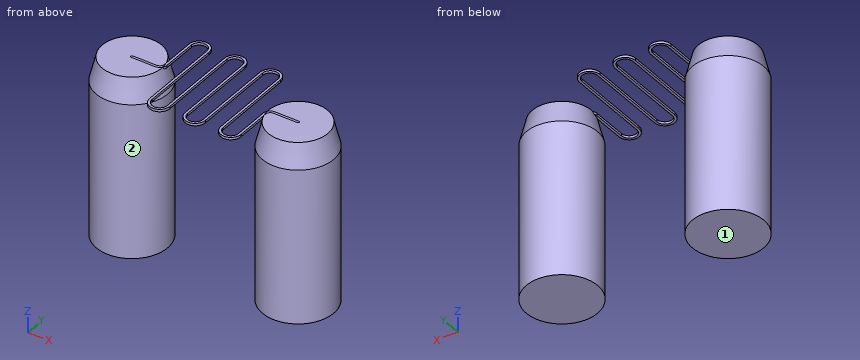
```python
from build123d import *
from build123d.topology import SkipClean

# Parameters (mm, degrees)
BOSS_EXTRUDE1_DEPTH = 0.4


with BuildPart() as part:
    # Sketch2 → Boss-Extrude1 (new body)
    with BuildSketch(Plane.XY):
        with BuildLine():
            Line((-17.5, -0.2), (-13.5, -0.2))
            ThreePointArc((-13.5, -0.2), (-12.651471863, 0.151471863), (-12.3, 1))
            Line((-12.3, 1), (-12.3, 7))
            ThreePointArc((-12.3, 7), (-11, 8.3), (-9.7, 7))
            Line((-9.7, 7), (-9.7, 0))
            Line((-9.7, 0), (-9.7, -7))
            ThreePointArc((-9.7, -7), (-8, -8.7), (-6.3, -7))
            Line((-6.3, -7), (-6.3, 0))
            Line((-6.3, 0), (-6.3, 7))
            ThreePointArc((-6.3, 7), (-5, 8.3), (-3.7, 7))
            Line((-3.7, 7), (-3.7, 0))
            Line((-3.7, 0), (-3.7, -7))
            ThreePointArc((-3.7, -7), (-2, -8.7), (-0.3, -7))
            Line((-0.3, -7), (-0.3, 0))
            Line((-0.3, 0), (-0.3, 7))
            ThreePointArc((-0.3, 7), (1, 8.3), (2.3, 7))
            Line((2.3, 7), (2.3, 0))
            Line((2.3, 0), (2.3, -7))
            ThreePointArc((2.3, -7), (4, -8.7), (5.7, -7))
            Line((5.7, -7), (5.7, -1))
            ThreePointArc((5.7, -1), (5.934314575, -0.434314575), (6.5, -0.2))
            Line((6.5, -0.2), (10.5, -0.2))
            ThreePointArc((10.5, -0.2), (10.7, 0), (10.5, 0.2))
            Line((10.5, 0.2), (6.5, 0.2))
            ThreePointArc((6.5, 0.2), (5.651471863, -0.151471863), (5.3, -1))
            Line((5.3, -1), (5.3, -7))
            ThreePointArc((5.3, -7), (4, -8.3), (2.7, -7))
            Line((2.7, -7), (2.7, 0))
            Line((2.7, 0), (2.7, 7))
            ThreePointArc((2.7, 7), (1, 8.7), (-0.7, 7))
            Line((-0.7, 7), (-0.7, 0))
            Line((-0.7, 0), (-0.7, -7))
            ThreePointArc((-0.7, -7), (-2, -8.3), (-3.3, -7))
            Line((-3.3, -7), (-3.3, 0))
            Line((-3.3, 0), (-3.3, 7))
            ThreePointArc((-3.3, 7), (-5, 8.7), (-6.7, 7))
            Line((-6.7, 7), (-6.7, 0))
            Line((-6.7, 0), (-6.7, -7))
            ThreePointArc((-6.7, -7), (-8, -8.3), (-9.3, -7))
            Line((-9.3, -7), (-9.3, 0))
            Line((-9.3, 0), (-9.3, 7))
            ThreePointArc((-9.3, 7), (-11, 8.7), (-12.7, 7))
            Line((-12.7, 7), (-12.7, 1))
            ThreePointArc((-12.7, 1), (-12.934314575, 0.434314575), (-13.5, 0.2))
            Line((-13.5, 0.2), (-17.5, 0.2))
            ThreePointArc((-17.5, 0.2), (-17.7, 0), (-17.5, -0.2))
        make_face()
    extrude(amount=BOSS_EXTRUDE1_DEPTH)

    # Sketch3 → Revolve1 (revolve)
    with SkipClean():  # the faces are left unmerged after this step: merging them gives an invalid solid
        with BuildSketch(Plane(origin=(0, 0, 0), x_dir=(-1, 0, 0), z_dir=(0, -1, 0)), mode=Mode.PRIVATE) as revolve1_sk:
            Polygon((17.5, -0.4), (22.5, -0.4), (23.5, 3.6), (23.5, 29.6), (17.5, 29.6), align=None)
        revolve(revolve1_sk.sketch.rotate(Axis((-17.5, 0, 0.4), (0, 0, -1)), 160.250078189), axis=Axis((-17.5, 0, 0.4), (0, 0, -1)))

    # Sketch4 → Revolve2 (revolve)
    with SkipClean():  # the faces are left unmerged after this step: merging them gives an invalid solid
        with BuildSketch(Plane(origin=(0, 0, 0), x_dir=(-1, 0, 0), z_dir=(0, -1, 0)), mode=Mode.PRIVATE) as revolve2_sk:
            Polygon((-10.5, -0.4), (-15.5, -0.4), (-16.5, 3.6), (-16.5, 29.6), (-10.5, 29.6), align=None)
        revolve(revolve2_sk.sketch.rotate(Axis((10.5, 0, 0.4), (0, 0, -1)), 176.315074658), axis=Axis((10.5, 0, 0.4), (0, 0, -1)))


solid = part.part
```
Design review of the part built by this model. Coordinates are the model's own, in mm. Face numbers are marked on the shaded views. Give positions to 0.01 mm unless a question says otherwise; leave off trailing zeros. Loops run counter-clockwise (first coordinate to the right, second up) from the corner with the lowest first, then second, coordinate; pieces in that order, holes last. Notation, with made-up numbers: M -34,22.25 L 19,22.25 A29 cw 19,47.25 Z; hole C 59.25,-35 d11. An arc over 180 degrees is marked long. Return JSON: item names as keys, results as strings. Group by question number.
Item 1: We need section A-A (x = 1). Give the boundary of the cut face in (y, z).
Item 2: Insertion check: pin 1 Ø3 at (x, y) = (-11.5, -5.5) entering from +Z; pin 2 Ø4 at (x, y) = (-6.5, 5.5) entering from -Z; pin 3 Ø3 at (y, z) = (-3, -13) entering from -X; pin 4 Ø3 at (y, z) = (-5.5, -7) entering from +X. Each pin has a flat end and moves straight along its axis. Give the tip position at first contact, or say it passes through.
Item 3: We need section C-C (y = 3.75). Give the number of separate pieces and of enclosed holes in the cut face, and give its area (3 significant figures).
Item 4: For probe 1 along X at (y, z) = (-0.25, -14); probe 2 along Z at (x, y) = (-9.5, 2.25); probe 3 along X at (y, z) = (3.5, -27), list the stretches that pass through material, from the lowest coordinate up.
Item 5: We need section B-B (z = -7.5). Give the boundary of the cut face in (x, y).
Item 6: Mouldability with a two-part tool opening along X and no side actions: class the marked faces 1 and 2 as released by +X, released by -X, zero draft, split by the parting line, or undercut.
Output:
{
 "1": {"outline": "M 8.3,0 L 8.7,0 L 8.7,0.4 L 8.3,0.4 Z"},
 "2": {"pin 1": "passes through", "pin 2": "stops at z = 0", "pin 3": "stops at x = -23.31", "pin 4": "stops at x = 14.97"},
 "3": {"separate pieces": "8", "enclosed holes": "0", "area": "552 mm^2"},
 "4": {"probe 1": "x = -23.49 to -11.51, 4.51 to 16.49", "probe 2": "z = 0 to 0.4", "probe 3": "x = -22.37 to -12.63, 5.63 to 15.37"},
 "5": {"outline": "C -17.5,0 d12; C 10.5,0 d12"},
 "6": {"face 1": "zero draft", "face 2": "undercut"}
}
